Model file for the job. Use its own axes, mm. Face numbers are marked on the shaded views. A direction names the side the tool comes from. Give positions to 0.01 mm unless a question says otherwise; leave off trailing zeros. Loops run counter-clockwise (first coordinate to the right, second up) from the corner with the lowest first, then second, coordinate; pieces in that order, holes last. Notation, with made-up numbers: M -24,76.5 L 8,76.5 A26 ccw 8,102.5 Z; hole C 63,65.25 d6. An arc over 180 degrees is marked long. Answer in a Markdown table with one row per item.
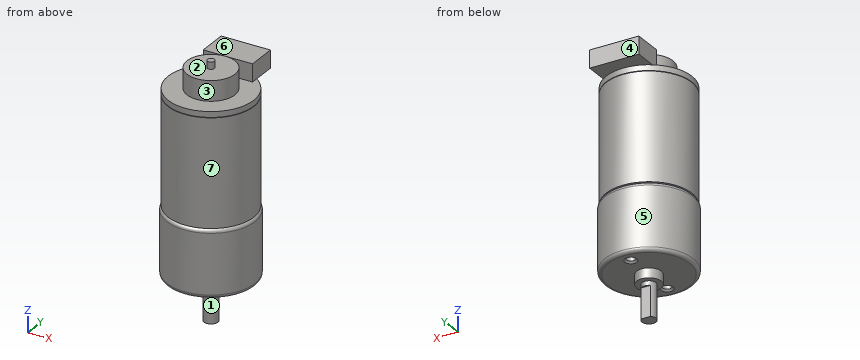
Autodesk Inventor part; units mm, degrees
ref_plane "YZ Plane" through (0, 0, 0) normal (1, 0, 0) x (0, 1, 0)
ref_plane "XZ Plane" through (0, 0, 0) normal (0, 1, 0) x (-1, 0, 0)
ref_plane "XY Plane" through (0, 0, 0) normal (0, 0, 1) x (1, 0, 0)
sketch "Эскиз1" plane through (0, 0, 0) normal (1, 0, 0) x (0, 1, 0)
  line L0 (0, 0) -> (11.15, 0)
  line L1 (12.15, 0.134) -> (12.15, 30.616)
  line L2 (12.15, 30.75) -> (11.65, 30.75)
  line L3 (11.65, 30.75) -> (12.15, 30.616)
  line L4 (11.65, 30.75) -> (12.7154, 30.75) construction
  line L5 (12.15, 30.75) -> (12.15, 32.35)
  line L6 (12.15, 32.35) -> (0, 32.35)
  line L7 (11.65, 30.75) -> (0, 30.75)
  line L8 (0, 32.35) -> (0, 0)
  line L9 (12.15, 0) -> (11.65, 0)
  line L10 (11.65, 0) -> (12.15, 0.134)
  line L11 (0, 32.35) -> (6.8, 32.35)
  line L12 (6.8, 32.35) -> (6.8, 38.05)
  line L13 (6.8, 38.05) -> (0, 38.05)
  line L14 (0, 38.05) -> (0, 32.35)
  line L15 (0, 38.05) -> (0, 40.05)
  line L16 (0, 40.05) -> (1, 40.05)
  line L17 (1, 40.05) -> (1, 38.05)
  line L18 (11.65, 0) -> (12.15, 0)
  line L19 (0, 0) -> (0, -19)
  line L20 (0, -19) -> (0, -21.75)
  line L21 (0, -21.75) -> (3.5, -21.75)
  line L22 (3.5, -21.75) -> (3.5, -19)
  line L23 (0, -21.75) -> (2, -21.75)
  line L24 (2, -21.75) -> (2, -31.55)
  line L25 (2, -31.55) -> (0, -31.55)
  line L26 (0, -31.55) -> (0, -21.75)
  line L27 (11.65, 0) -> (11.15, 0)
  line L28 (0, -19) -> (11.5, -19)
  line L29 (12.5, -18) -> (12.5, -1)
  line L30 (11.5, 0) -> (11.65, 0)
  arc A0 (12.5, -1) -> (11.5, 0) centre (11.5, -1) ccw
  arc A1 (11.5, -19) -> (12.5, -18) centre (11.5, -18) ccw
  point P0 (12.5, -19)
  dimension "d0" = 12.15
  dimension "d1" = 30.75
  dimension "d2" = 0.5
  dimension "d4" = 15
  dimension "d5" = 1.6
  dimension "d6" = 0.5
  dimension "d7" = 15
  dimension "d8" = 6.8
  dimension "d9" = 5.7
  dimension "d10" = 2
  dimension "d11" = 1
  dimension "d13" = 2.75
  dimension "d14" = 3.5
  dimension "d15" = 2
  dimension "d16" = 9.8
  dimension "d23" = 12.5
  dimension "d24" = 1
revolve "Вращение1" add sketch "Эскиз1" angle 360 about axis through (0, 0, 38.05) along (0, 0, 1) contours L15 L16 L17 L13
revolve "Вращение2" add sketch "Эскиз1" angle 360 about axis through (0, 0, 38.05) along (0, 0, -1) contours L14 L13 L12 L6
revolve "Вращение3" add sketch "Эскиз1" angle 360 about axis through (0, 0, 32.35) along (0, 0, -1) contours L8 L6 L5 L2 L7
revolve "Вращение4" add sketch "Эскиз1" angle 360 about axis through (0, 0, 32.35) along (0, 0, -1) contours L8 L7 L3 L1 L10 L27 L0
revolve "Вращение5" add sketch "Эскиз1" angle 360 about axis through (0, 0, 0) along (0, 0, -1) contours L0 L27 A0 L29 A1 L28 L19
revolve "Вращение6" add sketch "Эскиз1" angle 360 about axis through (0, 0, -19) along (0, 0, -1) contours L28 L22 L21 L20
revolve "Вращение7" add sketch "Эскиз1" angle 360 about axis through (0, 0, -31.55) along (0, 0, 1) contours L21 L24 L25 L26
sketch "Эскиз2" plane through (0, 0, 32.35) normal (0, 0, 1) x (1, 0, 0)
  line L0 (-7, 7.95) -> (7, 7.95)
  line L1 (7, 7.95) -> (7, 16.35)
  line L2 (7, 16.35) -> (-7, 16.35)
  line L3 (-7, 16.35) -> (-7, 7.95)
  line L4 (-7, 7.95) -> (7, 16.35) construction
  line L5 (7, 7.95) -> (-7, 16.35) construction
  circle A0 centre (0, 0) radius 12.15
  point P0 (0, 12.15)
  dimension "d28" = 14
  dimension "d29" = 8.4
extrude "Выдавливание1" add sketch "Эскиз2" along normal blind 5 contours L3 A0 L1 L0 | L3 L2 L1 A0 picked at (-0.4961, 9.3195)
sketch "Эскиз3" plane through (0, 0, -31.55) normal (0, 0, -1) x (-1, 0, 0)
  line L0 (-1.8903, 1.5) -> (1.8903, 1.5)
  line L1 (1.8903, 1.5) -> (1.8903, 3.1362)
  line L2 (1.8903, 3.1362) -> (-1.8903, 3.1362)
  line L3 (-1.8903, 3.1362) -> (-1.8903, 1.5)
  line L4 (-1.8903, 1.5) -> (1.8903, 3.1362) construction
  line L5 (1.8903, 1.5) -> (-1.8903, 3.1362) construction
  circle A0 centre (0, 0) radius 2
  point P0 (0, 2.3181)
  dimension "d32" = 1.5
extrude "Выдавливание2" cut sketch "Эскиз3" against normal blind 8.55 contours L3 L2 L1 L0 A0 | A0 L0 picked at (0, 1.6667)
sketch "Эскиз4" plane through (0, 0, -19) normal (0, 0, -1) x (-1, 0, 0)
  circle A0 centre (0, 0) radius 3.5
  circle A1 centre (0, 0) radius 11.5
  circle A2 centre (0, 8.5) radius 0.4758
  line L0 (-17.5, 0) -> (17.5, 0)
  circle A3 centre (0, -8.5) radius 0.4758
  dimension "d35" = 8.5
hole "Отверстие1" at (0, 8.5, -19) at (0, -8.5, -19) direction (0, 0, 1) diameter 2.459 depth 11.5 tip angle 118 countersink diameter 3.5 countersink angle 90
properties part number "servo"
(1) Saw through at B-B, the plane z = -10. Give the cut face in (x, y).
Established:
| item | result |
|---|---|
| outline | C 0,0 d25; hole C 0,-8.5 d2.46; hole C 0,8.5 d2.46 |
(2) Which spindle directions (+Z, -Z, +X, -X, +Y, -Y) get a long thin tool onto all of the face, cutting with end or side? Do the marked faces 4, 5, 6 and 7. Say none if no direction does.
Established:
| item | result |
|---|---|
| face 4 | +Z, -Z, +X, -X, +Y |
| face 5 | -Z |
| face 6 | +Z, +X, -X, +Y |
| face 7 | none |
(3) Wall check: L1, parallel to Z at x = -4.5, y = 3; L2, parallel to Z at x = 2, y = -7; L3, parallel to X at y = -8.5, z = -13. Give the ranges that are in metal, low to high.
Established:
| item | result |
|---|---|
| L1 | z = -19 to 38.05 |
| L2 | z = -19 to 32.35 |
| L3 | x = -9.17 to -1.23, 1.23 to 9.17 |
(4) Saw through at A-A, the plane z = 35. Give the cut face in (x, y), and give its area (3 significant figures).
Established:
| item | result |
|---|---|
| outline | M -7,7.95 L 7,7.95 L 7,16.35 L -7,16.35 Z; C 0,0 d13.6 |
| area | 263 mm2 |
(5) Saw through at C-C, the plane z = -2.5. Give the cut face in (x, y).
Established:
| item | result |
|---|---|
| outline | C 0,0 d25 |
(6) Flat gauge pins, fed straight in: P1, Ø1, axis at x = 5.5, z = 22.5, coming from the +Y side; P2, Ø2, axis at y = 11.5, z = 0.5, coming from the +X side; P3, Ø5, axis at x = 3, z = 14.5, coming from the +Y side. Where does each tip first touch, or does it go through?
Established:
| item | result |
|---|---|
| P1 | stops at y = 11.07 |
| P2 | stops at x = 6.11 |
| P3 | stops at y = 12.14 |
(7) Mould opens along Y. For the marked faces 1, 2 and 3 say: pulls with the +Y half, pulls with the -Y half, needs draft (parallel to the pull), parting line crosses it, or undercut.
Established:
| item | result |
|---|---|
| face 1 | parting line crosses it |
| face 2 | needs draft |
| face 3 | undercut |
(8) Saw through at D-D, the plane z = 19. Give the cut face in (x, y).
Established:
| item | result |
|---|---|
| outline | C 0,0 d24.3 |
